```python
from build123d import *

# Parameters (mm, degrees)
BOSS_EXTRUDE2_DEPTH = 38.1
SKETCH7_W           = 6.35
SKETCH7_H           = 50.8
CUT_EXTRUDE1_DEPTH  = 25.4
SKETCH8_R           = 7.62
CUT_EXTRUDE3_DEPTH  = 53.34


with BuildPart() as part:
    # Sketch3 → Boss-Extrude2 (new, symmetric)
    with BuildSketch(Plane.XY):
        Polygon((0, 18.396289168), (0, -45.103710832), (38.1, -83.203710832), (88.9, -83.203710832), (88.9, -57.803710832), (69.85, -57.803710832), (69.85, -32.403710832), (44.45, -7.003710832), (25.4, -7.003710832), (25.4, 18.396289168), align=None)
    extrude(amount=BOSS_EXTRUDE2_DEPTH, both=True)

    # Sketch7 → Cut-Extrude1 (cut)
    with BuildSketch(Plane(origin=(0, 18.396289168, 0), x_dir=(1, 0, 0), z_dir=(0, 1, 0))):
        with Locations((22.225, 0)):
            Rectangle(SKETCH7_W, SKETCH7_H)
    extrude(amount=-CUT_EXTRUDE1_DEPTH, mode=Mode.SUBTRACT)

    # Sketch8 → Cut-Extrude3 (cut)
    with BuildSketch(Plane(origin=(18.723144584, 18.723144584, 0), x_dir=(0, 0, -1), z_dir=(0.7071067811865487, 0.7071067811865465, 0))):
        with Locations(Location((-19.05, -54.346492331, 0), (0, 0, 90))):
            Circle(SKETCH8_R)
        with Locations(Location((19.05, -54.346492331, 0), (0, 0, 90))):
            Circle(SKETCH8_R)
    extrude(amount=-CUT_EXTRUDE3_DEPTH, mode=Mode.SUBTRACT)


solid = part.part
```
Build history of the part. All positions in model axes, mm. A direction names the side the tool comes from. Give positions to 0.01 mm unless a question says otherwise; leave off trailing zeros. Loops run counter-clockwise (first coordinate to the right, second up) from the corner with the lowest first, then second, coordinate; pieces in that order, holes last. Notation, with made-up numbers: (-7, 37) - (17, 37) arc R16 cw to (17, 51) - close; hole circle Ø10 at (-23, 33). An arc over 180 degrees is marked (long way). Use a Markdown table: item, result.
(1) Drop flat-ended pins along their axis: pin 1 Ø9.5 at (x, z) = (81, 6.5) entering from +Y; pin 2 Ø4 at (y, z) = (5, -34) entering from +X; pin 3 Ø7.5 at (x, z) = (26.5, -14) entering from +Y. Give the stop position or say it passes through.
Taken from the geometry:
| item | result |
|---|---|
| pin 1 | y = -57.8 |
| pin 2 | x = 25.4 |
| pin 3 | y = -7 |
(2) Which spindle directions (+Z, -Z, +X, -X, +Y, -Y) get a long thin tool onto all of the face, cutting with end or side? Do faces 5 (the face through (25.4, 6, -32)), 6 (the face through (19.05, 6, 0)), 7 (the face through (0, -13, 1)), 8 (the face through (19.51, -57.5, 19.16)), 9 (the face through (34, -43, 38.1)). Say none if no direction does.
Taken from the geometry:
| item | result |
|---|---|
| face 5 | +Z, -Z, +X, +Y |
| face 6 | +X, +Y |
| face 7 | +Z, -Z, -X, +Y, -Y |
| face 8 | none |
| face 9 | +Z, +X, -X, +Y, -Y |
(3) Band-saw the part on C-C (y = -60.5). Give the number of separate pieces and of enclosed holes in the cut face, and give its area (3 significant figures).
Taken from the geometry:
| item | result |
|---|---|
| separate pieces | 1 |
| enclosed holes | 2 |
| area | 5,520 mm2 |
(4) Band-saw the part on D-D (z = 3). Give the cut face in (x, y), and give its area (3 significant figures).
Taken from the geometry:
| item | result |
|---|---|
| outline | (0, -45.1) - (38.1, -83.2) - (88.9, -83.2) - (88.9, -57.8) - (69.85, -57.8) - (69.85, -32.4) - (44.45, -7) - (19.05, -7) - (19.05, 18.4) - (0, 18.4) - close |
| area | 5,240 mm2 |
(5) Pull direction Z, two halves, no side cores. Call faces 1 (the face through (32, -7.004, 1)), 2 (the face through (34, -43, -38.1)), 3 (the face through (39.725, -39.468, -26.489)), 4 (the face through (69.85, -45, 1)): +Z half, -Z half, draft (parallel to the pull), parting line (faces both ways), or undercut.
Taken from the geometry:
| item | result |
|---|---|
| face 1 | undercut |
| face 2 | -Z half |
| face 3 | undercut |
| face 4 | draft |
(6) Band-saw the part on B-B (x = 72). Give the cut face in (y, z), and give its area (3 significant figures).
Taken from the geometry:
| item | result |
|---|---|
| outline | (-83.2, -38.1) - (-57.8, -38.1) - (-57.8, 38.1) - (-83.2, 38.1) - close |
| area | 1,940 mm2 |
(7) Band-saw the part on A-A (z = -24). Give the cut face in (x, y), and give its area (3 significant figures).
Taken from the geometry:
| item | result |
|---|---|
| outline | (0, -45.1) - (38.1, -83.2) - (88.9, -83.2) - (88.9, -57.8) - (69.85, -57.8) - (69.85, -32.4) - (61.25, -23.8) - (23.53, -61.52) - (15.34, -53.33) - (53.06, -15.61) - (44.45, -7) - (19.05, -7) - (19.05, 18.4) - (0, 18.4) - close |
| area | 4,620 mm2 |
(8) Wall check: line 1 along Z through (x, y) = (54, -18.5); line 2 along Z through (x, y) = (34, -46); line 3 along Y through (x, z) = (80, 0). Give the ranges that are in metal, low to high.
Taken from the geometry:
| item | result |
|---|---|
| line 1 | -38.1 to -26.02, -12.08 to 12.08, 26.02 to 38.1 |
| line 2 | -38.1 to -26.34, -11.76 to 11.76, 26.34 to 38.1 |
| line 3 | -83.2 to -57.8 |
